Design review of the part shown in the three views and the two pictorial views. Dimensions are in mm from the part's minimum x, y and z. A direction names the side the tool comes from. Round coordinates to 2 decimals unless told otherwise and drop trailing zeros. Order: outer loops, then holes, each group sorted by start corner. A loop starts at its lowest first (then second) coordinate and runs counter-clockwise, first axis right, second up.
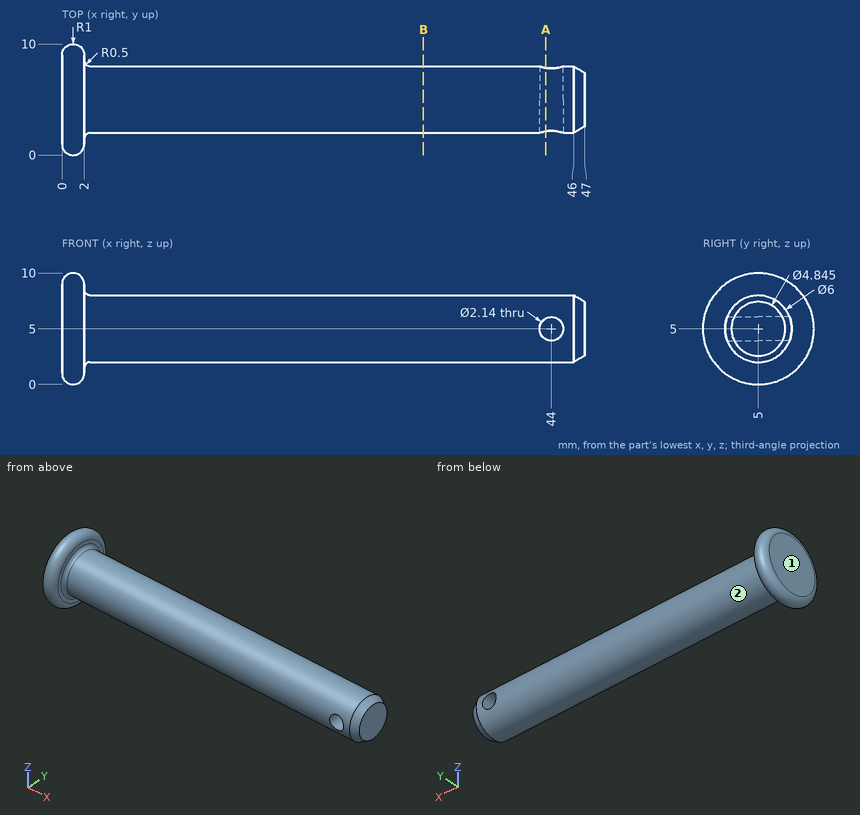
1) Clearance check with flat-ended pins moving along their axes: P1, Ø6, axis at x = 24, y = 3, coming from the +Z side; P2, Ø2, axis at y = 9, z = 7, coming from the +X side; P3, Ø6, axis at x = 10, y = 1, coming from the +Z side. State where each tip first meets the part, or that it passes through.
Results:
P1: stops at z = 8
P2: stops at x = 2
P3: stops at z = 7.83
2) Take a section at B-B on x = 32.5. Give the boundary of the cut face in (y, z).
Results:
outline: circle Ø6 at (5, 5)
3) Take a section at A-A on x = 43.5. Give the boundary of the cut face in (y, z), plus the area to 3 significant figures.
Results:
outline: (2.15, 4.05) arc R3 ccw to (7.85, 4.05) - close; (2.15, 5.95) - (7.85, 5.95) arc R3 ccw to start
area: 17.1 mm2
4) For the marked faces 1 and 2, list the 3-axis set-ups (+Z, -Z, +X, -X, +Y, -Y) from which the entire face can be reached by the end or side of a thin tool; tool diameter is ignored.
Results:
face 1: +Z, -Z, -X, +Y, -Y
face 2: +X
5) To check wall thickness, follow line 1 along Z through (x, y) = (44, 7.3) (1 decimal); line 2 along X through (y, z) = (4.5, 9); line 3 along Z through (x, y) = (44, 3.6). State the ranges of each line that lie inside material, in increasing order.
Results:
line 1: z = 3.1 to 3.9, 6.1 to 6.9
line 2: x = 0 to 2
line 3: z = 2.35 to 3.93, 6.07 to 7.65
